Autodesk Inventor part; units mm, degrees
ref_plane "YZ Plane" through (0, 0, 0) normal (1, 0, 0) x (0, 1, 0)
ref_plane "XZ Plane" through (0, 0, 0) normal (0, 1, 0) x (-1, 0, 0)
ref_plane "XY Plane" through (0, 0, 0) normal (0, 0, 1) x (1, 0, 0)
sketch "Szkic1" plane through (0, 0, 0) normal (0, 1, 0) x (-1, 0, 0)
  line L0 (-2.5, -5) -> (2.5, -5)
  line L1 (2.5, -5) -> (2.5, 5)
  line L2 (2.5, 5) -> (-2.5, 5)
  line L3 (-2.5, 5) -> (-2.5, -5)
  line L4 (-2.5, -5) -> (2.5, 5) construction
  line L5 (2.5, -5) -> (-2.5, 5) construction
  point P0 (0, 0)
  dimension "d0" = 5
  dimension "d1" = 10
extrude "Wyciągnięcie proste1" add sketch "Szkic1" along normal mid plane 94
sketch "Szkic3" plane through (2.5, -47, 5) normal (1, 0, 0) x (0, 0, -1)
  circle A0 centre (5, 5) radius 2.75
  line L0 (10, 0) -> (0, 0)
  line L1 (10, 0) -> (10, 94)
  point P0 (5, 47)
  point P1 (10, 118)
  dimension "d10" = 5.5
  dimension "d11" = 5
  dimension "d12" = 5
extrude "Wyciągnięcie proste3" cut sketch "Szkic3" against normal blind 120
sketch "Szkic4" plane through (2.5, -47, -5) normal (1, 0, 0) x (0, 0, -1)
  point P0 (-5, 47)
sketch "Szkic5" plane through (0, 47, 0) normal (0, 1, 0) x (1, 0, 0)
  line L0 (5, -5) -> (-5, -5)
  line L1 (-5, -5) -> (-5, 5)
  line L2 (-5, 5) -> (5, 5)
  line L3 (5, 5) -> (5, -5)
  line L4 (5, -5) -> (-5, 5) construction
  line L5 (-5, -5) -> (5, 5) construction
  point P0 (0, 0)
  dimension "d16" = 10
  dimension "d17" = 10
extrude "Wyciągnięcie proste4" add sketch "Szkic5" against normal blind 20
sketch "Szkic6" plane through (5, 47, 5) normal (1, 0, 0) x (0, 0, -1)
  circle A0 centre (5, -5) radius 2.75
  line L0 (0, 0) -> (10, 0)
  line L1 (0, 0) -> (0, -20)
  point P0 (5, -47)
  dimension "d20" = 5.5
  dimension "d21" = 5
  dimension "d22" = 5
extrude "Wyciągnięcie proste5" cut sketch "Szkic6" against normal blind 20
fillet "Zaokrąglenie3" radius 2 6 edges at (2.5, 27, 0) (5, 27, 0) (-5, 27, 0) (-2.5, 27, 0) (-5, 47, 0) (5, 47, 0)
properties part number "element_posredni"
Source: CAD feature listing. Evaluate the final solid. Frame: model axes, mm. A direction names the side the tool comes from. Coordinates: 2 decimals unless noted, no trailing zeros. Order: outer loops, then holes, each group sorted by start corner. A loop starts at its lowest first (then second) coordinate and runs counter-clockwise, first axis right, second up.
Item 1: Cut plane A-A (y = -42). Return loops of the section in (x, z).
Output values:
outline: (-2.5, -5) - (2.5, -5) - (2.5, -2.75) - (-2.5, -2.75) - close; (-2.5, 2.75) - (2.5, 2.75) - (2.5, 5) - (-2.5, 5) - close
Item 2: Cut plane C-C (y = 42). Return loops of the section in (x, z).
Output values:
outline: (-5, -5) - (5, -5) - (5, -2.75) - (-5, -2.75) - close; (-5, 2.75) - (5, 2.75) - (5, 5) - (-5, 5) - close
Item 3: Cut plane B-B (x = -1.25). Return loops of the section in (y, z), plus the area to 3 significant figures.
Output values:
outline: (-47, -5) - (47, -5) - (47, 5) - (-47, 5) - close; hole circle Ø5.5 at (-42, 0); hole circle Ø5.5 at (42, 0)
area: 892 mm2
Item 4: Material intervals for line 1 (Y direction, x = -1, z = 0); line 2 (X direction, y = 3, z = -0.75); line 3 (Y direction, x = 4.5, z = -0.5), sorted ascending.
Output values:
line 1: y = -47 to -44.75, -39.25 to 39.25, 44.75 to 47
line 2: x = -2.5 to 2.5
line 3: y = 27.39 to 39.3, 44.7 to 46.32
Item 5: Set-up query: faces 4 (the face through (-2.5, -12, 0)), 5 (the face through (5, 35, 0)). Return all of +Z, -Z, +X, -X, +Y, -Y with unobstructed straight access to the full face (end or side cutting, diameter ignored); none if empty.
Output values:
face 4: +Z, -Z, -X, -Y
face 5: +Z, -Z, +X, +Y, -Y
Item 6: Cut plane D-D (z = 0). Count the separate pieces of the cut face and the enclosed holes in it, plus the area to 3 significant figures.
Output values:
separate pieces: 3
enclosed holes: 0
area: 487 mm2
Item 7: Pull-direction query (Z, two-part tool) for faces 1 (the face through (0, 11, -5)), 2 (the face through (0.07, 44.727, 0.358)), 3 (the face through (2.5, -12, 0)); classes: pulls with the +Z half, pulls with the -Z half, needs draft (parallel to the pull), parting line crosses it, or undercut.
Output values:
face 1: pulls with the -Z half
face 2: undercut
face 3: needs draft
Item 8: First-contact query: P1, Ø5, axis at y = -23.5, z = 1.5, coming from the +X side; P2, Ø1, axis at y = -1.5, z = -2, coming from the -X side. Flat tips, straight axial feed; report the tip coordinate or a pass-through.
Output values:
P1: stops at x = 2.5
P2: stops at x = -2.5
